Input: dimensioned drawing with shaded views. Units: mm. Origin: part minimum x, y, z. A direction names the side the tool comes from. Give positions to 0.01 mm unless a question says otherwise; leave off trailing zeros. Order: outer loops, then holes, each group sorted by start corner. A loop starts at its lowest first (then second) coordinate and runs counter-clockwise, first axis right, second up.
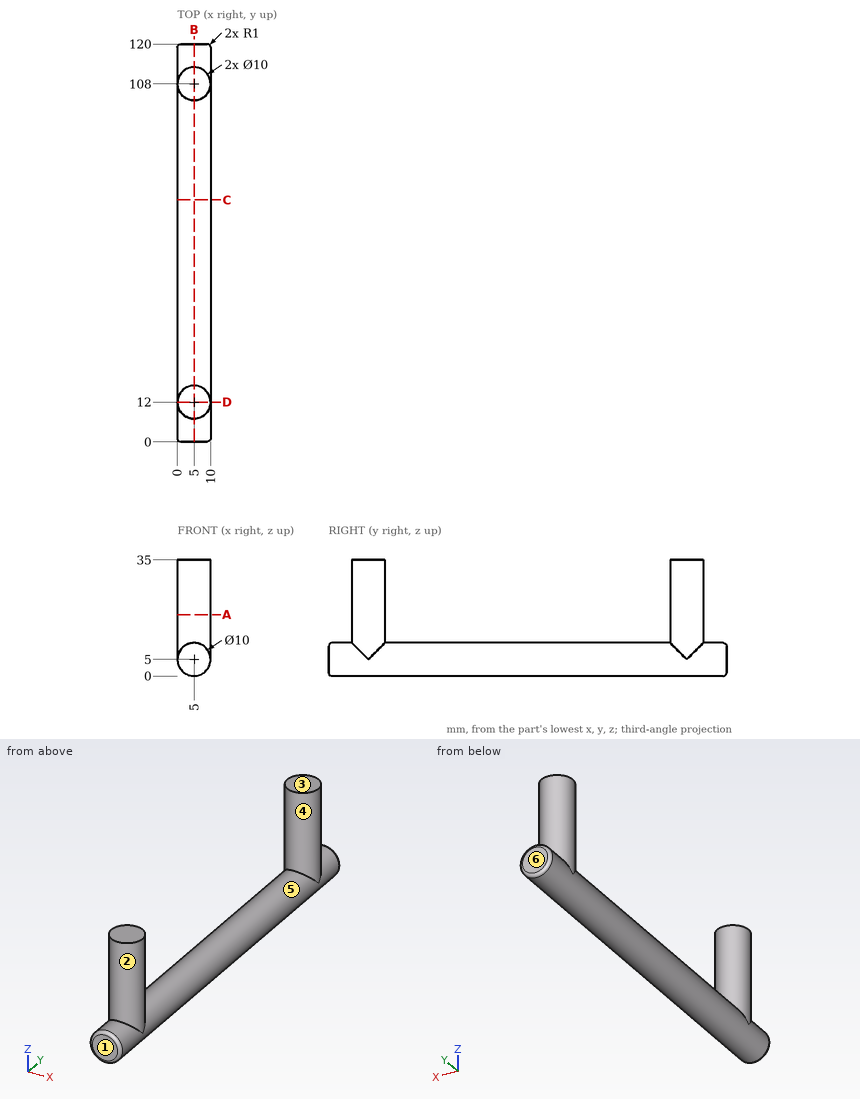
1) Material intervals for L1, parallel to Z at x = 8, y = 7.5; L2, parallel to Y at x = 9.25, z = 32; L3, parallel to Y at x = 5.75, z = 13, sorted ascending.
Report:
L1: z = 1 to 9
L2: y = 9.37 to 14.63, 105.37 to 110.63
L3: y = 7.06 to 16.94, 103.06 to 112.94
2) Draft query along Y for the marked faces 1, 2 and 3. Return one class per face: +Y half, -Y half, draft (parallel to the pull), parting line (faces both ways), or undercut.
Report:
face 1: -Y half
face 2: undercut
face 3: draft
3) Section query C-C, the plane y = 73. Return the cut outline in (x, z), and give its area (3 significant figures).
Report:
outline: circle Ø10 at (5, 5)
area: 78.5 mm2
4) Reachability of the marked faces 4, 5 and 6 from +Z, -Z, +X, -X, +Y, -Y: full face, straight path, thin tool, end or side. Return the list, or none.
Report:
face 4: +Z
face 5: none
face 6: +Z, -Z, +X, -X, +Y
5) Section query A-A, the plane z = 18.5. Return the cut outline in (x, y).
Report:
outline: circle Ø10 at (5, 12); circle Ø10 at (5, 108)
6) Section query D-D, the plane y = 12. Return the cut outline in (x, z), and give its area (3 significant figures).
Report:
outline: (0, 5) arc R5 ccw to (10, 5) - (10, 35) - (0, 35) - close
area: 339 mm2
7) Pin query (flat end, axial travel): pin 1 (6 mm diameter, centred on x = 3.5, z = 26.5, fed in from +Y); pin 2 (5 mm diameter, centred on x = 6.5, z = 27, fed in from -Y); pin 3 (1.5 mm diameter, centred on x = 3, z = 24.5, fed in from +Y). Return the tip coordinate at first contact, or that it passes through.
Report:
pin 1: stops at y = 113
pin 2: stops at y = 7
pin 3: stops at y = 112.84
8) Section query B-B, the plane x = 5. Return the cut outline in (y, z), and give its area (3 significant figures).
Report:
outline: (0, 1) arc R1 ccw to (1, 0) - (119, 0) arc R1 ccw to (120, 1) - (120, 9) arc R1 ccw to (119, 10) - (113, 10) - (113, 35) - (103, 35) - (103, 10) - (17, 10) - (17, 35) - (7, 35) - (7, 10) - (1, 10) arc R1 ccw to (0, 9) - close
area: 1,700 mm2
